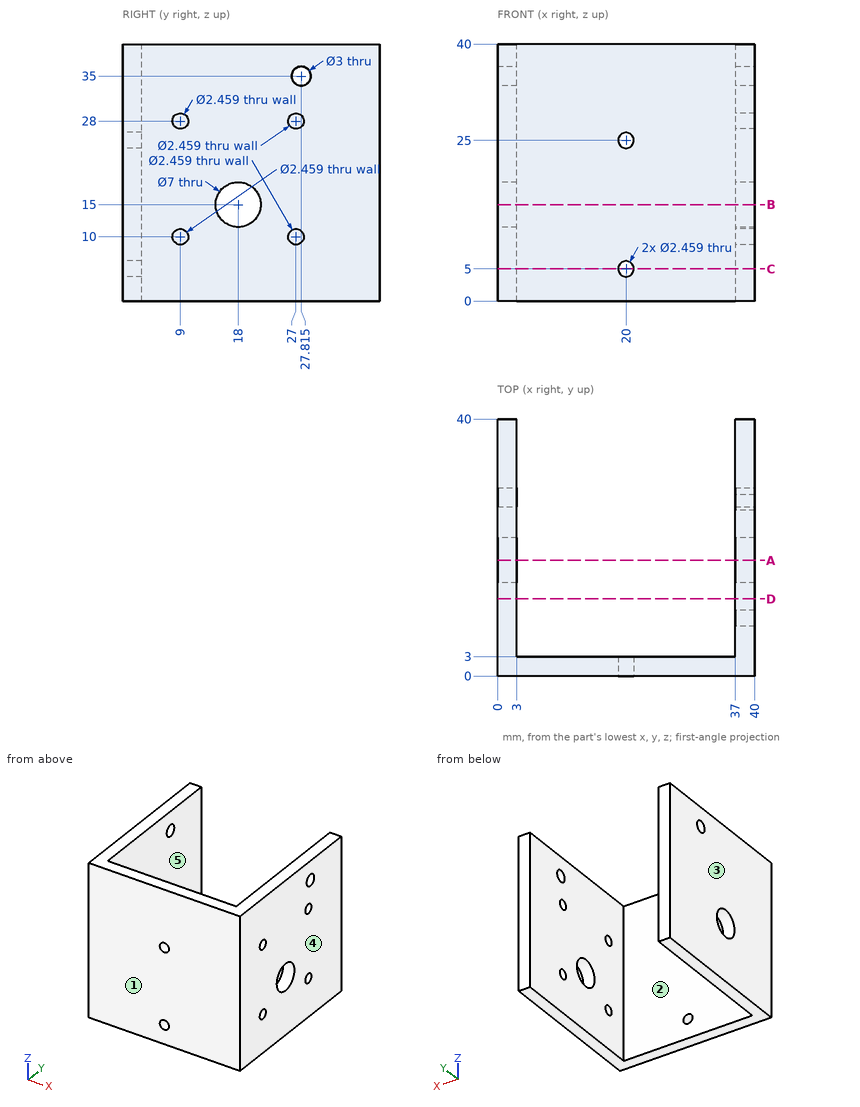
For this review, use the dimensioned drawing (mm, ordinates from the lowest corner) and the shaded views. A direction names the side the tool comes from. Round coordinates to 2 decimals unless told otherwise and drop trailing zeros. Loops run counter-clockwise (first coordinate to the right, second up) from the corner with the lowest first, then second, coordinate; pieces in that order, holes last. Notation, with made-up numbers: M -2.5,67 L 26.5,67 A4 cw 26.5,71 Z; hole C 3,53.25 d5. An arc over 180 degrees is marked long. Answer as CSV lines item,"result".
1. Draft analysis for pull direction X (two halves, no side actions). For the marked faces 3, 4 and 5, state which applies: pulls with the +X half, pulls with the -X half, needs draft (parallel to the pull), parting line crosses it, or undercut.
Outcome:
face 3,"pulls with the -X half"
face 4,"pulls with the +X half"
face 5,"undercut"
2. We need section D-D (y = 12). Give the boundary of the cut face in (x, z), plus the area to 3 significant figures.
Outcome:
outline,"M 0,0 L 3,0 L 3,40 L 0,40 Z; M 37,0 L 40,0 L 40,40 L 37,40 Z"
area,"240 mm2"
3. Insertion check: pin 1 Ø1.8 at (y, z) = (27.81, 35) entering from +X; pin 2 Ø1.5 at (y, z) = (9, 28) entering from +X; pin 3 Ø4 at (x, z) = (18, 13.5) entering from +Y. Each pin has a flat end and moves straight along its axis. Give the tip position at first contact, or say it passes through.
Outcome:
pin 1,"passes through"
pin 2,"stops at x = 3"
pin 3,"stops at y = 3"
4. For the marked faces 1 and 2, list the 3-axis set-ups (+Z, -Z, +X, -X, +Y, -Y) from which the entire face can be reached by the end or side of a thin tool; tool diameter is ignored.
Outcome:
face 1,"+Z, -Z, +X, -X, -Y"
face 2,"+Z, -Z, +Y"
5. To check wall thickness, follow L1, parallel to Z at x = 20, y = 0.7; L2, parallel to X at y = 32, z = 20; L3, parallel to Y at x = 2, z = 15. State the ranges of each line that lie inside material, in increasing order. Write a range as [from, to].
Outcome:
L1,"z = [0, 3.77], [6.23, 23.77], [26.23, 40]"
L2,"x = [0, 3], [37, 40]"
L3,"y = [0, 14.5], [21.5, 40]"
6. We need section A-A (y = 18). Give the boundary of the cut face in (x, z).
Outcome:
outline,"M 0,0 L 3,0 L 3,11.5 L 0,11.5 Z; M 0,18.5 L 3,18.5 L 3,40 L 0,40 Z; M 37,0 L 40,0 L 40,11.5 L 37,11.5 Z; M 37,18.5 L 40,18.5 L 40,40 L 37,40 Z"
7. We need section B-B (z = 15). Give the boundary of the cut face in (x, y), plus the area to 3 significant figures.
Outcome:
outline,"M 0,0 L 40,0 L 40,14.5 L 37,14.5 L 37,3 L 3,3 L 3,14.5 L 0,14.5 Z; M 0,21.5 L 3,21.5 L 3,40 L 0,40 Z; M 37,21.5 L 40,21.5 L 40,40 L 37,40 Z"
area,"300 mm2"
8. We need section C-C (z = 5). Give the boundary of the cut face in (x, y), plus the area to 3 significant figures.
Outcome:
outline,"M 0,0 L 18.77,0 L 18.77,3 L 3,3 L 3,40 L 0,40 Z; M 21.23,0 L 40,0 L 40,40 L 37,40 L 37,3 L 21.23,3 Z"
area,"335 mm2"
